For this review, take the finished solid that the model builds, in its own axes (mm). Coordinates: 2 decimals unless noted, no trailing zeros. Write each loop counter-clockwise with the first axis right and the second up, starting at its lowest first coordinate (ties: lowest second). Pieces come first, ordered by that corner, then holes.
```python
from build123d import *

# Parameters (mm, degrees)
F0_R     = 35.5
F0_R_2   = 33.5
F1_DEPTH = 50.8
F3_R     = 13
F4_DEPTH = 44.45
F6_DEPTH = 38.1


with BuildPart() as f1:
    # F0 (on Front) → F1 (new body)
    with BuildSketch(Plane.XZ):
        Circle(F0_R)
        Circle(F0_R_2, mode=Mode.SUBTRACT)
    extrude(amount=F1_DEPTH)

    # F3 (on offset) → F4 (cut)
    with BuildSketch(Plane.XY.offset(38.1)):
        with BuildLine():
            ThreePointArc((5.538755, -28.298548), (-24.386056, -26.798548), (5.538755, -25.298548))
            Line((5.538755, -25.298548), (15.851872, -25.298548))
            Line((15.851872, -25.298548), (15.851872, -20.093698))
            Line((15.851872, -20.093698), (18.351872, -20.093698))
            Line((18.351872, -20.093698), (18.351872, -25.298548))
            Line((18.351872, -25.298548), (35.634305, -25.298548))
            Line((35.634305, -25.298548), (35.634305, 3.781537))
            Line((35.634305, 3.781537), (-42.059839, 3.781537))
            Line((-42.059839, 3.781537), (-40.54736, -55.053797))
            Line((-40.54736, -55.053797), (35.634305, -53.095396))
            Line((35.634305, -53.095396), (35.634305, -28.298548))
            Line((35.634305, -28.298548), (18.351872, -28.298548))
            Line((18.351872, -28.298548), (18.351872, -33.503398))
            Line((18.351872, -33.503398), (15.851872, -33.503398))
            Line((15.851872, -33.503398), (15.851872, -28.298548))
            Line((15.851872, -28.298548), (5.538755, -28.298548))
        make_face()
        with Locations((-9.386056, -26.798548)):
            Circle(F3_R)
    extrude(amount=-F4_DEPTH, mode=Mode.SUBTRACT)

    # F5 (on Right) → F6 (cut, symmetric)
    with BuildSketch(Plane.YZ):
        Polygon((-28.453713, -37.598766), (-28.453713, -6.049039), (-52.303165, -5.728194), (-52.303165, -37.598766), align=None)
        Polygon((4.118928, -6.049039), (-25.245266, -6.049039), (-25.245266, -37.270404), (5.401779, -37.682697), align=None)
    extrude(amount=F6_DEPTH, both=True, mode=Mode.SUBTRACT)


solid = f1.part
```
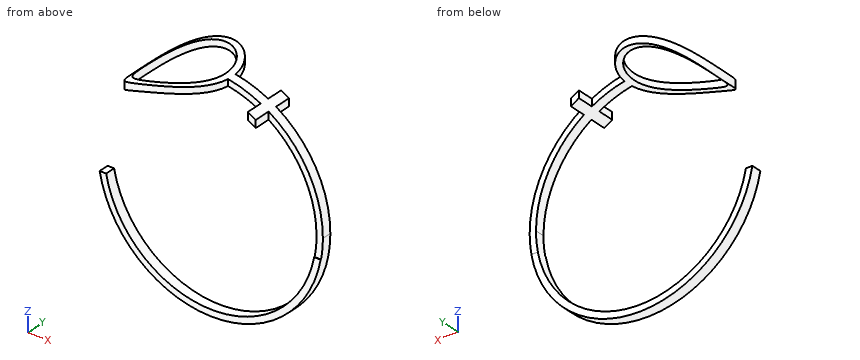
Q1. For probe 1 along X at (y, z) = (-27, -22.5); probe 2 along Y at (x, z) = (24, -26); probe 3 along X at (y, z) = (-22.5, 27), list the stretches that pass through material, from the lowest coordinate up.
Ans:
probe 1: x = -27.46 to -24.82, 24.82 to 27.46
probe 2: y = -28.45 to -25.25
probe 3: x = -23.05 to -21.65
Q2. Clearance check with flat-ended pins moving along their axes: pin 1 Ø4.5 at (x, z) = (9, 31.5) entering from +Y; pin 2 Ø8 at (y, z) = (-19.5, 10.5) entering from -X; pin 3 Ø3 at (x, z) = (17.5, 30.5) entering from +Y; pin 4 Ø1.9 at (y, z) = (-30, 28.5) entering from +X. State where each tip first meets the part, or that it passes through.
Ans:
pin 1: stops at y = -25.3
pin 2: passes through
pin 3: stops at y = -20.09
pin 4: stops at x = 18.35
Q3. Add section B-B (x = 31.5). State the section outline as (y, z) points.
Ans:
outline: (-28.45, -16.37) - (-25.25, -16.37) - (-25.25, -11.4) - (-28.45, -11.4) - close; (-28.3, 11.4) - (-25.3, 11.4) - (-25.3, 16.37) - (-28.3, 16.37) - close
Q4. Add section A-A (y = -23). State the section outline as (x, z) points (3 decimals), then the cut area to 3 significant figures.
Ans:
outline: (-23.897, 23.477) arc R33.5 cw to (-21.819, 25.42) - (-21.819, 28.003) arc R35.5 ccw to (-23.897, 26.252) - close; (3.047, 33.361) arc R33.5 cw to (5.125, 33.106) - (5.125, 35.128) arc R35.5 ccw to (3.047, 35.369) - close; (15.852, 29.512) arc R33.5 cw to (18.352, 28.026) - (18.352, 30.388) arc R35.5 ccw to (15.852, 31.764) - close
area: 15.5 mm2
Q5. Add section D-D (x = -16). State the section outline as (y, z) points, then the cut area to 3 significant figures.
Ans:
outline: (-40.26, 29.43) - (-37.99, 29.43) - (-37.99, 31.69) - (-40.26, 31.69) - close; (-28.45, -31.69) - (-25.25, -31.69) - (-25.25, -29.43) - (-28.45, -29.43) - close; (-15.61, 29.43) - (-13.34, 29.43) - (-13.34, 31.69) - (-15.61, 31.69) - close
area: 17.5 mm2
Q6. Add section C-C (z = -8). State the section outline as (x, y) points.
Ans:
outline: (-34.59, -28.45) - (-32.53, -28.45) - (-32.53, -25.25) - (-34.59, -25.25) - close; (32.53, -28.45) - (34.59, -28.45) - (34.59, -25.25) - (32.53, -25.25) - close
